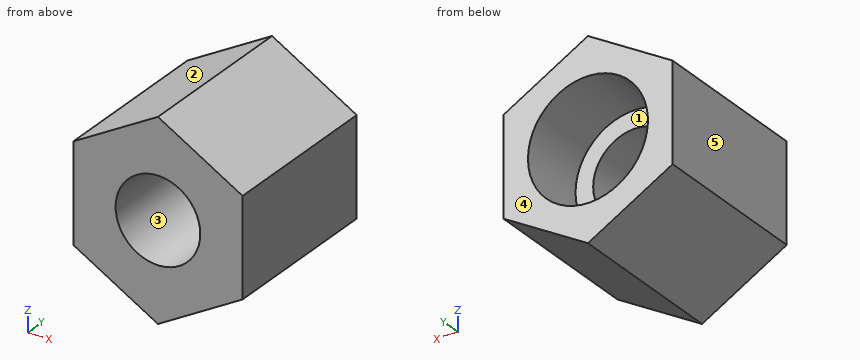
```python
from build123d import *

# Parameters (mm, degrees)
SKETCH_1_R          = 6
EXTRUDE_1_DEPTH     = 24
SKETCH_3_R          = 8.5
CUT_EXTRUDE_2_DEPTH = 10


with BuildPart() as part:
    # Эскиз1 → Бобышка-Вытянуть1 (new body)
    with BuildSketch(Plane(origin=(0, 0, 0), x_dir=(1, 0, 0), z_dir=(0, 1, 0))):
        Polygon((0, 13.856406461), (-12, 6.92820323), (-12, -6.92820323), (0, -13.856406461), (12, -6.92820323), (12, 6.92820323), align=None)
        Circle(SKETCH_1_R, mode=Mode.SUBTRACT)
    extrude(amount=EXTRUDE_1_DEPTH)

    # Эскиз3 → Вырез-Вытянуть2 (cut)
    with BuildSketch(Plane(origin=(0, 24, 0), x_dir=(1, 0, 0), z_dir=(0, 1, 0))):
        Circle(SKETCH_3_R)
    extrude(amount=-CUT_EXTRUDE_2_DEPTH, mode=Mode.SUBTRACT)


solid = part.part
```
Input: part model. Units: mm. Frame: model coordinates. Face numbers are marked on the shaded views. A direction names the side the tool comes from. Give positions to 0.01 mm unless a question says otherwise; leave off trailing zeros. Order: outer loops, then holes, each group sorted by start corner. A loop starts at its lowest first (then second) coordinate and runs counter-clockwise, first axis right, second up. Notation, with made-up numbers: (-9.75, 79) - (31.25, 79) arc R21 cw to (31.25, 114) - close; hole circle Ø4 at (68, 61.5). An arc over 180 degrees is marked (long way). Put each result on its own line as item: value.
Item 1: Contact query for flat-ended pins moving along their axis: pin 1 (8.5 mm diameter, centred on x = -0.5, z = 4, fed in from +Y); pin 2 (3 mm diameter, centred on x = 6, y = 6, fed in from -Z); pin 3 (1 mm diameter, centred on y = 9.5, z = -7.5, fed in from +X). Output: stop coordinate, or through.
Found:
pin 1: stops at y = 14
pin 2: stops at z = -11.26
pin 3: stops at x = 11.88
Item 2: Section query B-B, the plane y = 9.25. Return loops of the section in (x, z).
Found:
outline: (-12, -6.93) - (0, -13.86) - (12, -6.93) - (12, 6.93) - (0, 13.86) - (-12, 6.93) - close; hole circle Ø12 at (0, 0)
Item 3: Access query for the marked faces 1 and 2. Directions: +Z, -Z, +X, -X, +Y, -Y. A direction counts if a zero-diameter tool reaches every point of the face in a straight line with its end or side. Return the directions, or none.
Found:
face 1: +Y
face 2: +Z, -X, +Y, -Y
Item 4: Section query C-C, the plane x = -2.25. Return loops of the section in (y, z).
Found:
outline: (0, -12.56) - (24, -12.56) - (24, -8.2) - (14, -8.2) - (14, -5.56) - (0, -5.56) - close; (0, 5.56) - (14, 5.56) - (14, 8.2) - (24, 8.2) - (24, 12.56) - (0, 12.56) - close
Item 5: Draft query along X for the marked faces 3, 4 and 5. Return one class per face: +X half, -X half, draft (parallel to the pull), parting line (faces both ways), or undercut.
Found:
face 3: undercut
face 4: draft
face 5: -X half
Item 6: Ray query, L1, parallel to X at y = 7.25, z = 0; L2, parallel to X at y = 16.75, z = 0; L3, parallel to Z at x = 0, y = 4.5. Return the intervals inside material, ascending. Write a range as from..to.
Found:
L1: x = -12..-6, 6..12
L2: x = -12..-8.5, 8.5..12
L3: z = -13.86..-6, 6..13.86
Item 7: Section query D-D, the plane y = 15.5. Return loops of the section in (x, z).
Found:
outline: (-12, -6.93) - (0, -13.86) - (12, -6.93) - (12, 6.93) - (0, 13.86) - (-12, 6.93) - close; hole circle Ø17 at (0, 0)
Item 8: Section query A-A, the plane z = 0. Return loops of the section in (x, y), then the cut area to 3 significant figures.
Found:
outline: (-12, 0) - (-6, 0) - (-6, 14) - (-8.5, 14) - (-8.5, 24) - (-12, 24) - close; (6, 0) - (12, 0) - (12, 24) - (8.5, 24) - (8.5, 14) - (6, 14) - close
area: 238 mm^2
